Check sheet for the modelled part. Datum: model origin and axes. Units: mm. Face numbers are marked on the shaded views. Coordinates: 2 decimals unless noted, no trailing zeros. Order: outer loops, then holes, each group sorted by start corner. A loop starts at its lowest first (then second) coordinate and runs counter-clockwise, first axis right, second up.
1. Cross-section at C-C (y = 0). Enter the section's corners in (x, z), then the cut area to 3 significant figures.
2. Cross-section at B-B (x = -1). Enter the section's corners in (y, z).
3. Thickness scan on line 1 (Z direction, x = -26, y = -3.5); line 2 (Z direction, x = 16, y = -14); line 3 (X direction, y = 2.5, z = -12). Record the ranges inside material, lowest first.
4. Draft check along X on the marked faces 1, 2 and 3. Enter one of: released by +X, released by -X, zero draft, split by the parting line, or undercut.
5. Cross-section at D-D (z = 6). Enter the section's corners in (x, y).
6. Cross-section at A-A (y = -17.5). Enter the section's corners in (x, z), then the cut area to 3 significant figures.
7. Gauge pin test, flat ends, axial feed: pin 1 Ø10 at (x, y) = (19, 1) entering from +Z; pin 2 Ø14.5 at (y, z) = (7.5, -10) entering from -X; pin 3 Ø10 at (x, y) = (-12.5, 14) entering from -Z; pin 4 Ø7 at (x, y) = (0, -3.5) entering from -Z. Record the tip position at first contact, or that the pin passes through.
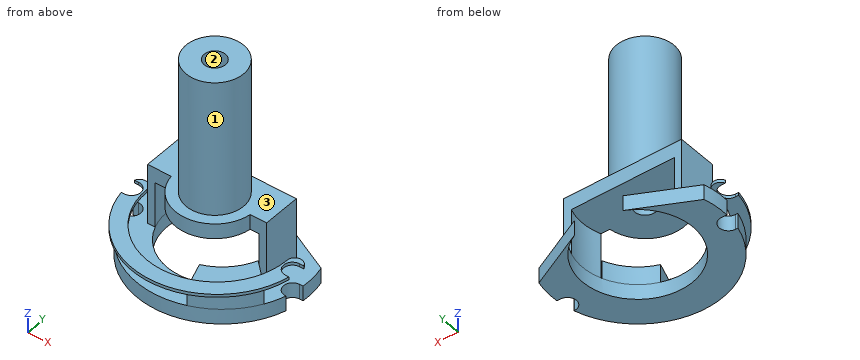
```python
from build123d import *

# Parameters (mm, degrees)
CROQUIS1_R              = 9.5
SALIENTE_EXTRUIR1_DEPTH = 45
SALIENTE_EXTRUIR2_DEPTH = 5
CROQUIS3_W              = 2.5
CROQUIS3_H              = 12.459614936
CROQUIS3_H_2            = 13
SALIENTE_EXTRUIR3_DEPTH = 20
SALIENTE_EXTRUIR4_DEPTH = 5
CORTAR_EXTRUIR1_DEPTH   = 15
CORTAR_EXTRUIR2_DEPTH   = 15
SALIENTE_EXTRUIR6_DEPTH = 6
SALIENTE_EXTRUIR9_DEPTH = 1
CORTAR_EXTRUIR3_DEPTH   = 30
CORTAR_EXTRUIR4_DEPTH   = 30
CROQUIS14_R             = 3.5
CORTAR_EXTRUIR5_DEPTH   = 71


with BuildPart() as part:
    # Croquis1 → Saliente-Extruir1 (new body)
    with BuildSketch(Plane.XY):
        Circle(CROQUIS1_R)
    extrude(amount=SALIENTE_EXTRUIR1_DEPTH)

    # Croquis2 → Saliente-Extruir2 (add)
    with BuildSketch(Plane(origin=(0, 0, 0), x_dir=(-1, 0, 0), z_dir=(0, 0, -1))):
        with BuildLine():
            Line((-13.86026331, 10.949878275), (16.13973669, 10.949878275))
            Line((16.13973669, 10.949878275), (18.13973669, 10.949878275))
            Line((18.13973669, 10.949878275), (18.13973669, -2.050121725))
            Line((18.13973669, -2.050121725), (12.837328418, -2.050121725))
            ThreePointArc((12.837328418, -2.050121725), (-0.272762426, -12.997138172), (-12.912036834, -1.509736661))
            Line((-12.912036834, -1.509736661), (-15.86026331, -1.509736661))
            Line((-15.86026331, -1.509736661), (-15.86026331, 10.949878275))
            Line((-15.86026331, 10.949878275), (-13.86026331, 10.949878275))
        make_face()
    extrude(amount=SALIENTE_EXTRUIR2_DEPTH)

    # Croquis3 → Saliente-Extruir3 (add)
    with BuildSketch(Plane.XY):
        with Locations((17.11026331, 4.720070807)):
            Rectangle(CROQUIS3_W, CROQUIS3_H)
        with Locations((-19.38973669, 4.449878275)):
            Rectangle(CROQUIS3_W, CROQUIS3_H_2)
    extrude(amount=-SALIENTE_EXTRUIR3_DEPTH)

    # Croquis4 → Saliente-Extruir4 (add)
    with BuildSketch(Plane(origin=(0, 0, -20), x_dir=(-1, 0, 0), z_dir=(0, 0, -1))):
        with BuildLine():
            Line((-26.12024366, 11.549093047), (-6.789040969, 21.054674019))
            ThreePointArc((-6.789040969, 21.054674019), (1.243045599, -13.482502548), (9.275132167, 21.054674019))
            Line((9.275132167, 21.054674019), (28.606334858, 11.549093047))
            ThreePointArc((28.606334858, 11.549093047), (1.243045599, -23.482502548), (-26.12024366, 11.549093047))
        make_face()
    extrude(amount=SALIENTE_EXTRUIR4_DEPTH)

    # Croquis5 → Cortar-Extruir1 (cut)
    with BuildSketch(Plane(origin=(0, 0, -20), x_dir=(-1, 0, 0), z_dir=(0, 0, -1))):
        with BuildLine():
            Line((-15.86026331, 10.949878275), (-15.86026331, -1.509736661))
            ThreePointArc((-15.86026331, -1.509736661), (-16.959527756, 4.720070807), (-15.86026331, 10.949878275))
        make_face()
    extrude(amount=-CORTAR_EXTRUIR1_DEPTH, mode=Mode.SUBTRACT)

    # Croquis6 → Cortar-Extruir2 (cut)
    with BuildSketch(Plane(origin=(0, 0, -20), x_dir=(-1, 0, 0), z_dir=(0, 0, -1))):
        with BuildLine():
            Line((18.13973669, -2.050121725), (18.13973669, 10.949878275))
            Line((18.13973669, 10.949878275), (18.346354508, 10.949878275))
            ThreePointArc((18.346354508, 10.949878275), (19.443320322, 4.430801495), (18.13973669, -2.050121725))
        make_face()
    extrude(amount=-CORTAR_EXTRUIR2_DEPTH, mode=Mode.SUBTRACT)

    # Croquis8 → Saliente-Extruir6 (add)
    with BuildSketch(Plane.XY.offset(-20)):
        with BuildLine():
            Line((23.380531683, -9.030005034), (15.754093987, -1.793831452))
            ThreePointArc((15.754093987, -1.793831452), (11.418506022, -8.357344354), (4.718355695, -12.478631799))
            Line((4.718355695, -12.478631799), (7.993387845, -21.927132443))
            ThreePointArc((7.993387845, -21.927132443), (16.873495336, -16.894185793), (23.380531683, -9.030005034))
        make_face()
    extrude(amount=SALIENTE_EXTRUIR6_DEPTH)

    # Croquis10 → Saliente-Extruir9 (add)
    with BuildSketch(Plane.XY.offset(-14)):
        with BuildLine():
            ThreePointArc((-29.094443415, 2.096360018), (-0.89187006, -26.106213336), (27.310703295, 2.096360018))
            ThreePointArc((27.310703295, 2.096360018), (24.810703295, 4.596360018), (22.310703295, 2.096360018))
            ThreePointArc((22.310703295, 2.096360018), (-0.89187006, -21.106213336), (-24.094443415, 2.096360018))
            ThreePointArc((-24.094443415, 2.096360018), (-26.594443415, 4.596360018), (-29.094443415, 2.096360018))
        make_face()
    extrude(amount=SALIENTE_EXTRUIR9_DEPTH)

    # Croquis12 → Cortar-Extruir3 (cut)
    with BuildSketch(Plane.XY.offset(-13)):
        with BuildLine():
            Line((-27.563915972, 3), (-28.925416341, 3))
            Line((-28.925416341, 3), (-33.584272261, 3))
            Line((-33.584272261, 3), (-33.584272261, -3))
            Line((-33.584272261, -3), (-28.63015152, -3))
            Line((-28.63015152, -3), (-27.563915972, -3))
            ThreePointArc((-27.563915972, -3), (-24.563915972, 0), (-27.563915972, 3))
        make_face()
    extrude(amount=-CORTAR_EXTRUIR3_DEPTH, mode=Mode.SUBTRACT)

    # Croquis13 → Cortar-Extruir4 (cut)
    with BuildSketch(Plane.XY.offset(-13)):
        with BuildLine():
            Line((25.714967949, 2.943204688), (33.854636773, 2.943204688))
            Line((33.854636773, 2.943204688), (33.854636773, -2.943204688))
            Line((33.854636773, -2.943204688), (25.714967949, -2.943204688))
            ThreePointArc((25.714967949, -2.943204688), (22.771763261, 0), (25.714967949, 2.943204688))
        make_face()
    extrude(amount=-CORTAR_EXTRUIR4_DEPTH, mode=Mode.SUBTRACT)

    # Croquis14 → Cortar-Extruir5 (cut, through all)
    with BuildSketch(Plane.XY.offset(45)):
        Circle(CROQUIS14_R)
    extrude(amount=-CORTAR_EXTRUIR5_DEPTH, mode=Mode.SUBTRACT)


solid = part.part
```
Data:
1. outline: (-24.56, -25) - (-18.82, -25) - (-18.82, -5) - (-3.5, -5) - (-3.5, 45) - (-9.5, 45) - (-9.5, 0) - (-20.64, 0) - (-20.64, -20) - (-24.56, -20) - close; (-24.56, -14) - (-24, -14) - (-24, -13) - (-24.56, -13) - close; (3.5, -5) - (16.34, -5) - (16.34, -25) - (22.77, -25) - (22.77, -20) - (18.36, -20) - (18.36, 0) - (9.5, 0) - (9.5, 45) - (3.5, 45) - close; (22.22, -14) - (22.77, -14) - (22.77, -13) - (22.22, -13) - close
1. area: 820 mm2
2. outline: (-26.11, -14) - (-21.11, -14) - (-21.11, -13) - (-26.11, -13) - close; (-23.48, -25) - (-13.48, -25) - (-13.48, -20) - (-23.48, -20) - close; (-12.96, -5) - (-3.35, -5) - (-3.35, 45) - (-9.45, 45) - (-9.45, 0) - (-12.96, 0) - close; (3.35, -5) - (10.95, -5) - (10.95, 0) - (9.45, 0) - (9.45, 45) - (3.35, 45) - close
3. line 1: z = -25 to -20, -14 to -13
3. line 2: z = -25 to -13
3. line 3: x = -20.64 to -19.31, 16.82 to 18.36
4. face 1: split by the parting line
4. face 2: undercut
4. face 3: zero draft
5. outline: circle Ø19 at (0, 0); hole circle Ø7 at (0, 0)
6. outline: (-21.17, -14) - (-13.32, -14) - (-13.32, -13) - (-21.17, -13) - close; (-18.61, -25) - (16.13, -25) - (16.13, -14) - (19.39, -14) - (19.39, -13) - (11.53, -13) - (11.53, -14) - (6.46, -14) - (6.46, -20) - (-18.61, -20) - close
6. area: 247 mm2
7. pin 1: stops at z = 0
7. pin 2: stops at x = -28.93
7. pin 3: stops at z = -25
7. pin 4: stops at z = -5
